```python
from build123d import *

# Parameters (mm, degrees)
SKETCH1_W           = 80
SKETCH1_H           = 25
BOSS_EXTRUDE1_DEPTH = 20
SKETCH3_W           = 76
SKETCH3_H           = 16
CUT_EXTRUDE1_DEPTH  = 23
SKETCH4_R           = 1
CUT_EXTRUDE2_DEPTH  = 48
SKETCH5_R           = 2.5
CUT_EXTRUDE3_DEPTH  = 48


with BuildPart() as part:
    # Sketch1 → Boss-Extrude1 (new body)
    with BuildSketch(Plane(origin=(0, 0, 0), x_dir=(1, 0, 0), z_dir=(0, 1, 0))):
        with Locations((-4.196598457, -17.578240617)):
            Rectangle(SKETCH1_W, SKETCH1_H)
    extrude(amount=BOSS_EXTRUDE1_DEPTH)

    # Sketch3 → Cut-Extrude1 (cut)
    with BuildSketch(Plane.XY.offset(30.078240617)):
        with Locations((-4.196598457, 10)):
            Rectangle(SKETCH3_W, SKETCH3_H)
    extrude(amount=-CUT_EXTRUDE1_DEPTH, mode=Mode.SUBTRACT)

    # Sketch4 → Cut-Extrude2 (cut)
    with BuildSketch(Plane.XY.offset(7.078240617)):
        with Locations((30.803401543, 10)):
            Circle(SKETCH4_R)
        with Locations((-39.196598457, 10)):
            Circle(SKETCH4_R)
    extrude(amount=-CUT_EXTRUDE2_DEPTH, mode=Mode.SUBTRACT)

    # Sketch5 → Cut-Extrude3 (cut)
    with BuildSketch(Plane.XY.offset(7.078240617)):
        with Locations((-31.696598457, 10)):
            Circle(SKETCH5_R)
        with Locations((23.303401543, 10)):
            Circle(SKETCH5_R)
    extrude(amount=-CUT_EXTRUDE3_DEPTH, mode=Mode.SUBTRACT)


solid = part.part
```
For this review, take the finished solid that the model builds, in its own axes (mm). A direction names the side the tool comes from. Coordinates: 2 decimals unless noted, no trailing zeros. Loops run counter-clockwise (first coordinate to the right, second up) from the corner with the lowest first, then second, coordinate; pieces in that order, holes last. Notation, with made-up numbers: (23, 30.5) -> (41, 30.5) arc R25 ccw to (41, 47.5) -> close; hole circle Ø5 at (-24, 22.5). An arc over 180 degrees is marked (long way). Return JSON: item names as keys, results as strings. Group by question number.
(1) Mouldability with a two-part tool opening along Y and no side actions: class faces 3 (the flat face through (-5, 0, 17)), 4 (the cylindrical face through (-39.93, 10.68, 6.09)), 5 (the flat face through (-5, 20, 17)) as pulls with the +Y half, pulls with the -Y half, needs draft (parallel to the pull), parting line crosses it, or undercut.
(2) Consider section C-C, the plane z = 24. Give the boundary of the cut face in (x, y), plus the area to 3 significant figures.
(3) To check wall thickness, follow L1, parallel to Y at x = -1.5, z = 14.25; L2, parallel to X at y = 3.5, z = 25; L3, parallel to Z at x = 9, y = 8. State the ranges of each line that lie inside material, in increasing order.
(4) Tool access review of faces 1 (the flat face through (-5, 18, 19)), 2 (the cylindrical face through (-34.194, 10.11, 6.092)): name each direction out of +Z, -Z, +X, -X, +Y, -Y from which nothing blocks a thin tool from reaching the whole face with its end or side.
(5) Consider section A-A, the plane y = 10. Give the boundary of the cut face in (x, z).
(6) Consider section D-D, the plane y = 6. Give the boundary of the cut face in (x, z), plus the area to 3 significant figures.
(7) For pin 1 Ø1 at (x, y) = (7.5, 10.5) entering from +Z; pin 2 Ø4 at (x, z) = (-30, 12.5) entering from -Y; pin 3 Ø3 at (x, y) = (-31.7, 10) entering from +Z, all flat-tipped, find the tip position at first contact; note any pin that passes through.
(8) Consider section B-B, the plane x = 3. Give the boundary of the cut face in (y, z), plus the area to 3 significant figures.
Results below:
{
 "1": {"face 3": "pulls with the -Y half", "face 4": "undercut", "face 5": "pulls with the +Y half"},
 "2": {"outline": "(-44.2, 0) -> (35.8, 0) -> (35.8, 20) -> (-44.2, 20) -> close; hole (-42.2, 2) -> (33.8, 2) -> (33.8, 18) -> (-42.2, 18) -> close", "area": "384 mm2"},
 "3": {"L1": "y = 0 to 2, 18 to 20", "L2": "x = -44.2 to -42.2, 33.8 to 35.8", "L3": "z = 5.08 to 7.08"},
 "4": {"face 1": "+Z", "face 2": "+Z, -Z"},
 "5": {"outline": "(-44.2, 5.08) -> (-40.2, 5.08) -> (-40.2, 7.08) -> (-42.2, 7.08) -> (-42.2, 30.08) -> (-44.2, 30.08) -> close; (-38.2, 5.08) -> (-34.2, 5.08) -> (-34.2, 7.08) -> (-38.2, 7.08) -> close; (-29.2, 5.08) -> (20.8, 5.08) -> (20.8, 7.08) -> (-29.2, 7.08) -> close; (25.8, 5.08) -> (29.8, 5.08) -> (29.8, 7.08) -> (25.8, 7.08) -> close; (31.8, 5.08) -> (35.8, 5.08) -> (35.8, 30.08) -> (33.8, 30.08) -> (33.8, 7.08) -> (31.8, 7.08) -> close"},
 "6": {"outline": "(-44.2, 5.08) -> (35.8, 5.08) -> (35.8, 30.08) -> (33.8, 30.08) -> (33.8, 7.08) -> (-42.2, 7.08) -> (-42.2, 30.08) -> (-44.2, 30.08) -> close", "area": "252 mm2"},
 "7": {"pin 1": "stops at z = 7.08", "pin 2": "stops at y = 0", "pin 3": "passes through"},
 "8": {"outline": "(0, 5.08) -> (20, 5.08) -> (20, 30.08) -> (18, 30.08) -> (18, 7.08) -> (2, 7.08) -> (2, 30.08) -> (0, 30.08) -> close", "area": "132 mm2"}
}
